Geometry: final body of the model. Coordinates: model frame, mm. A direction names the side the tool comes from. Round coordinates to 2 decimals unless told otherwise and drop trailing zeros. Loops run counter-clockwise (first coordinate to the right, second up) from the corner with the lowest first, then second, coordinate; pieces in that order, holes last. Notation, with made-up numbers: (36.25, 14) -> (94.25, 14) arc R27 cw to (94.25, 49) -> close; hole circle Ø6 at (-25.5, 61). An arc over 180 degrees is marked (long way). Answer in a Markdown table with one row per item.
```python
from build123d import *

# Parameters (mm, degrees)
F1_DEPTH = 30
F2_R     = 1.5
F3_DEPTH = 25


# Not quite as in the source:
# - a feature names something its author has since deleted; it is built from what else it names


with BuildPart() as f1:
    # F0 (on Front) → F1 (new body)
    with BuildSketch(Plane.XZ):
        Polygon((110, 150), (0, 0), (110, 0), align=None)
    extrude(amount=F1_DEPTH)

    # F2 (on face) → F3 (cut)
    with BuildSketch(Plane.YZ.offset(110)):
        with Locations((-15, 30)):
            Circle(F2_R)
        with Locations((-15, 60)):
            Circle(F2_R)
    extrude(amount=-F3_DEPTH, mode=Mode.SUBTRACT)


solid = f1.part
```
Item 1: Set-up query: faces 4 (the flat face through (110, -15, 74)), 5 (the flat face through (85, -15, 30)). Return all of +Z, -Z, +X, -X, +Y, -Y with unobstructed straight access to the full face (end or side cutting, diameter ignored); none if empty.
Ans:
| item | result |
|---|---|
| face 4 | +Z, -Z, +X, +Y, -Y |
| face 5 | +X |
Item 2: Section query B-B, the plane y = -27.5. Output: boundary loops of the cut face in (x, z).
Ans:
| item | result |
|---|---|
| outline | (0, 0) -> (110, 0) -> (110, 150) -> close |
Item 3: Section query C-C, the plane z = 11. Output: boundary loops of the cut face in (x, y).
Ans:
| item | result |
|---|---|
| outline | (8.07, -30) -> (110, -30) -> (110, 0) -> (8.07, 0) -> close |
Item 4: First-contact query: P1, Ø3, axis at x = 26, y = -3, coming from the +Z side; P2, Ø1.5, axis at y = -14.5, z = 60, coming from the +X side; P3, Ø10, axis at y = -13.5, z = 36, coming from the -X side. Flat tips, straight axial feed; report the tip coordinate or a pass-through.
Ans:
| item | result |
|---|---|
| P1 | z = 37.5 |
| P2 | x = 85 |
| P3 | x = 22.73 |
Item 5: Mould query, pull axis Z, two halves, no side actions, for faces 1 (the flat face through (54, -15, 0)), 2 (the flat face through (85, -15, 60)), 3 (the flat face through (79, 0, 43)). Classes: released by +Z, released by -Z, zero draft, split by the parting line, or undercut.
Ans:
| item | result |
|---|---|
| face 1 | released by -Z |
| face 2 | undercut |
| face 3 | zero draft |
Item 6: Ray query, L1, parallel to Z at x = 91, y = -15; L2, parallel to Z at x = 96, y = -15; L3, parallel to X at y = -22.25, z = 52.5. Return the intervals inside material, ascending.
Ans:
| item | result |
|---|---|
| L1 | 0 to 28.5, 31.5 to 58.5, 61.5 to 124.09 |
| L2 | 0 to 28.5, 31.5 to 58.5, 61.5 to 130.91 |
| L3 | 38.5 to 110 |
Item 7: Section query D-D, the plane x = 23. Output: boundary loops of the cut face in (y, z), and give its area (3 significant figures).
Ans:
| item | result |
|---|---|
| outline | (-30, 0) -> (0, 0) -> (0, 31.36) -> (-30, 31.36) -> close |
| area | 941 mm2 |
Item 8: Section query A-A, the plane x = 95.5. Output: boundary loops of the cut face in (y, z).
Ans:
| item | result |
|---|---|
| outline | (-30, 0) -> (0, 0) -> (0, 130.23) -> (-30, 130.23) -> close; hole circle Ø3 at (-15, 30); hole circle Ø3 at (-15, 60) |
